```python
from build123d import *

# Parameters (mm, degrees)
SKETCH1_R                                       = 20
BOSS_EXTRUDE1_DEPTH                             = 3.5
SKETCH4_R                                       = 23
BOSS_EXTRUDE2_DEPTH                             = 1
FILLET1_R                                       = 1
CSK_FOR_M3_FLAT_HEAD_MACHINE_SCREW1_D           = 3.4
CSK_FOR_M3_FLAT_HEAD_MACHINE_SCREW1_DEPTH       = 7
CSK_FOR_M3_FLAT_HEAD_MACHINE_SCREW1_CSINK_D     = 6.3
CSK_FOR_M3_FLAT_HEAD_MACHINE_SCREW1_CSINK_ANGLE = 90
CSK_FOR_M3_FLAT_HEAD_MACHINE_SCREW1_TIP         = 1.021463052
CUT_EXTRUDE1_DEPTH                              = 8


with BuildPart() as part:
    # Sketch1 → Boss-Extrude1 (new body, symmetric)
    with BuildSketch(Plane.XY):
        Circle(SKETCH1_R)
    extrude(amount=BOSS_EXTRUDE1_DEPTH, both=True)

    # Sketch3 → Revolve1 (revolve)
    with BuildSketch(Plane(origin=(0, 0, 0), x_dir=(1, 0, 0), z_dir=(0, 1, 0))):
        Polygon((-20, 3.5), (-23, 3.5), (-23, 3.3), (-20, 1.567949192), align=None)
    revolve(axis=Axis((0, 0, -3.5), (0, 0, 1)))

    # Sketch4 → Boss-Extrude2 (add)
    with BuildSketch(Plane.XY.offset(3.5)):
        Circle(SKETCH4_R)
    extrude(amount=-BOSS_EXTRUDE2_DEPTH)

    # Fillet1
    fillet1_edges = [part.edges().sort_by_distance(p)[0] for p in [
        (-20, 0, 2.5),
    ]]
    fillet(fillet1_edges, radius=FILLET1_R)

    # CSK for M3 Flat Head Machine Screw1
    with Locations(Plane(origin=(0, 0, -3.5), x_dir=(-1, 0, 0), z_dir=(0, 0, -1))):
        with Locations((0, 8), (-8, 0), (0, -8), (8, 0)):
            CounterSinkHole(CSK_FOR_M3_FLAT_HEAD_MACHINE_SCREW1_D / 2, CSK_FOR_M3_FLAT_HEAD_MACHINE_SCREW1_CSINK_D / 2, depth=CSK_FOR_M3_FLAT_HEAD_MACHINE_SCREW1_DEPTH, counter_sink_angle=CSK_FOR_M3_FLAT_HEAD_MACHINE_SCREW1_CSINK_ANGLE)
            with Locations((0, 0, -(CSK_FOR_M3_FLAT_HEAD_MACHINE_SCREW1_DEPTH + CSK_FOR_M3_FLAT_HEAD_MACHINE_SCREW1_TIP / 2))):  # 118° drill point
                Cone(0, CSK_FOR_M3_FLAT_HEAD_MACHINE_SCREW1_D / 2, CSK_FOR_M3_FLAT_HEAD_MACHINE_SCREW1_TIP, mode=Mode.SUBTRACT)

    # Sketch8 → Cut-Extrude1 (cut, through all)
    with BuildSketch(Plane(origin=(0, 0, -3.5), x_dir=(-1, 0, 0), z_dir=(0, 0, -1))):
        with BuildLine():
            Line((-1.5, 18.439088915), (-1.5, 12.409673646))
            ThreePointArc((-1.5, 12.409673646), (-4.783542905, 11.548494156), (-7.714304216, 9.835624559))
            Line((-7.714304216, 9.835624559), (-11.977744639, 14.099064982))
            ThreePointArc((-11.977744639, 14.099064982), (-7.079643499, 17.091771351), (-1.5, 18.439088915))
        make_face()
        with BuildLine():
            Line((1.5, 18.439088915), (1.5, 12.409673646))
            ThreePointArc((1.5, 12.409673646), (4.783542905, 11.548494156), (7.714304216, 9.835624559))
            Line((7.714304216, 9.835624559), (11.977744639, 14.099064982))
            ThreePointArc((11.977744639, 14.099064982), (7.079643499, 17.091771351), (1.5, 18.439088915))
        make_face()
        with BuildLine():
            Line((14.099064982, 11.977744639), (9.835624559, 7.714304216))
            ThreePointArc((9.835624559, 7.714304216), (11.548494156, 4.783542905), (12.409673646, 1.5))
            Line((12.409673646, 1.5), (18.439088915, 1.5))
            ThreePointArc((18.439088915, 1.5), (17.091771351, 7.079643499), (14.099064982, 11.977744639))
        make_face()
        with BuildLine():
            Line((18.439088915, -1.5), (12.409673646, -1.5))
            ThreePointArc((12.409673646, -1.5), (11.548494156, -4.783542905), (9.835624559, -7.714304216))
            Line((9.835624559, -7.714304216), (14.099064982, -11.977744639))
            ThreePointArc((14.099064982, -11.977744639), (17.091771351, -7.079643499), (18.439088915, -1.5))
        make_face()
        with BuildLine():
            Line((11.977744639, -14.099064982), (7.714304216, -9.835624559))
            ThreePointArc((7.714304216, -9.835624559), (4.783542905, -11.548494156), (1.5, -12.409673646))
            Line((1.5, -12.409673646), (1.5, -18.439088915))
            ThreePointArc((1.5, -18.439088915), (7.079643499, -17.091771351), (11.977744639, -14.099064982))
        make_face()
        with BuildLine():
            Line((-1.5, -18.439088915), (-1.5, -12.409673646))
            ThreePointArc((-1.5, -12.409673646), (-4.783542905, -11.548494156), (-7.714304216, -9.835624559))
            Line((-7.714304216, -9.835624559), (-11.977744639, -14.099064982))
            ThreePointArc((-11.977744639, -14.099064982), (-7.079643499, -17.091771351), (-1.5, -18.439088915))
        make_face()
        with BuildLine():
            Line((-14.099064982, -11.977744639), (-9.835624559, -7.714304216))
            ThreePointArc((-9.835624559, -7.714304216), (-11.548494156, -4.783542905), (-12.409673646, -1.5))
            Line((-12.409673646, -1.5), (-18.439088915, -1.5))
            ThreePointArc((-18.439088915, -1.5), (-17.091771351, -7.079643499), (-14.099064982, -11.977744639))
        make_face()
        with BuildLine():
            Line((-18.439088915, 1.5), (-12.409673646, 1.5))
            ThreePointArc((-12.409673646, 1.5), (-11.548494156, 4.783542905), (-9.835624559, 7.714304216))
            Line((-9.835624559, 7.714304216), (-14.099064982, 11.977744639))
            ThreePointArc((-14.099064982, 11.977744639), (-17.091771351, 7.079643499), (-18.439088915, 1.5))
        make_face()
    extrude(amount=-CUT_EXTRUDE1_DEPTH, mode=Mode.SUBTRACT)


solid = part.part
```
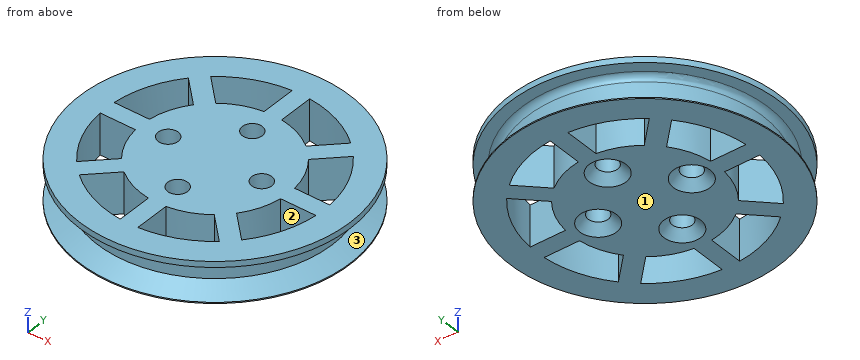
Can you work these out from the model? Positions are in its coordinate system, mm. Face numbers are marked on the shaded views. Round coordinates to 2 decimals unless told otherwise and drop trailing zeros. Loops run counter-clockwise (first coordinate to the right, second up) from the corner with the lowest first, then second, coordinate; pieces in that order, holes last. Notation, with made-up numbers: M -35.75,67.5 L -9.75,67.5 A32 ccw -9.75,104.5 Z; hole C 19,87 d2. An arc over 180 degrees is marked long. Write item = value, one per line. Start each with the question number.
(1) Suppose I cut it at C-C on z = 0.25. Give the number of separate pieces and of enclosed holes in the cut face, plus the area to 3 significant figures.
(2) If we mould it in two halves opening along Y, with no side actions, what happens to the marked faces 1, 2 and 3? For each: released by +Y, released by -Y, zero draft, split by the parting line, or undercut.
(3) I'm going to push flat-ended pins straight in: P1, Ø1.8, axis at y = 15.5, z = -0.5, coming from the -X side; P2, Ø23, axis at x = 11.5, y = 6, coming from the -Z side; P3, Ø1, axis at y = -7, z = 0.5, coming from the +X side; P4, Ø3, axis at x = 15, z = -1.5, coming from the +Y side. Where does each tip first touch, or does it pass through?
(4) Suppose I cut it at A-A on y = 0. Write out the boundary of the cut face in (x, z), plus the area to 3 significant figures.
(5) I need wall thicknesses on line 1 along Y through (x, z) = (0, -0.5); line 2 along Y through (x, z) = (-3, 2.75). Which ranges of each line are inside material? Lowest first, please.
Answer block:
q1.separate_pieces = 1
q1.enclosed_holes = 12
q1.area = 780 mm²
q2.face_1 = zero draft
q2.face_2 = undercut
q2.face_3 = split by the parting line
q3.P1 = -13.67
q3.P2 = -3.5
q3.P3 = 18.91
q3.P4 = 16.98
q4.outline = M -23,-3.5 L -11.15,-3.5 L -9.7,-2.05 L -9.7,3.5 L -23,3.5 L -23,2.5 L -21,2.5 A1 cw -20,1.5 L -20,-1.57 L -23,-3.3 Z; M -6.3,-2.05 L -4.85,-3.5 L 4.85,-3.5 L 6.3,-2.05 L 6.3,3.5 L -6.3,3.5 Z; M 9.7,-2.05 L 11.15,-3.5 L 23,-3.5 L 23,-3.3 L 20,-1.57 L 20,1.5 A1 cw 21,2.5 L 23,2.5 L 23,3.5 L 9.7,3.5 Z
q4.area = 241 mm²
q5.line_1 = -20 to -9.7, -6.3 to 6.3, 9.7 to 20
q5.line_2 = -22.8 to -18.26, -12.13 to 12.13, 18.26 to 22.8
